Input: part model. Units: mm. Frame: model coordinates. A direction names the side the tool comes from. Round coordinates to 2 decimals unless told otherwise and drop trailing zeros. Loops run counter-clockwise (first coordinate to the right, second up) from the corner with the lowest first, then second, coordinate; pieces in that order, holes last.
(1) Cut plane B-B, the plane y = 4.5. Output: boundary loops of the cut face in (x, z).
(2) Draft query along X for faces 1 (the face through (33.267, -9.491, -9.436)), 2 (the face through (64.422, 8, -4)), 3 (the face through (40.599, -5, -9)). Return one class per face: released by +X, released by -X, zero draft, split by the parting line, or undercut.
(3) First-contact query: pin 1 Ø6 at (x, z) = (59.5, -7.5) entering from -Y; pin 2 Ø1.5 at (x, y) = (44.5, 18.5) entering from +Z; pin 3 Ø1.8 at (y, z) = (-4, -9) entering from -X. Flat tips, straight axial feed; report the tip coordinate or a pass-through.
(4) Line query: line 1 (X direction, y = 4, z = -6.25); line 2 (Y direction, x = 51.5, z = -0.5); line 3 (Z direction, x = 31, y = 7). Output: solid intervals per line, ascending.
(5) Access query for faces 4 (the face through (44, -6.915, -9)), 5 (the face through (44.456, -9.419, -9.436)), 6 (the face through (33, -6.915, -9)), 7 (the face through (13.194, 8, -4)), 8 (the face through (39, -8, -7.62)). Directions: +Z, -Z, +X, -X, +Y, -Y. A direction counts if a zero-diameter tool reaches every point of the face in a straight line with its end or side. Return the directions, or none.
(6) Cut plane A-A, the plane z = -1. Output: boundary loops of the cut face in (x, y).
(7) Cut plane C-C, the plane x = 38.5. Output: boundary loops of the cut face in (y, z) (3 decimals), and give its area (3 significant figures).
(8) Cut plane D-D, the plane x = 30.5. Output: boundary loops of the cut face in (y, z) (3 decimals).
from build123d import *

# Parameters (mm, degrees)
BOSS_EXTRUDE4_DEPTH = 7.62
BOSS_EXTRUDE5_DEPTH = 3.5814
BOSS_EXTRUDE6_DEPTH = 3.5814


with BuildPart() as part:
    # Sketch17 → Boss-Extrude4 (new body)
    with BuildSketch(Plane(origin=(57.616701934, 0, 0), x_dir=(-1, 0, 0), z_dir=(0, 0, -1))):
        Polygon((-9.344833285, -2.54), (-9.344833285, 16.351663206), (2.490045751, 28.186542241), (34.995614796, 28.186542241), (46.962246821, 16.219910216), (46.962246821, -2.54), align=None)
        Polygon((-6.804833285, 0), (-6.804833285, 15.299560757), (3.542148199, 25.646542241), (33.943512348, 25.646542241), (44.422246821, 15.167807768), (44.422246821, 0), align=None, mode=Mode.SUBTRACT)
    extrude(amount=BOSS_EXTRUDE4_DEPTH)

    # Sketch20 → Boss-Extrude5 (add)
    with BuildSketch(Plane(origin=(0, 0, -7.62), x_dir=(-1, 0, 0), z_dir=(0, 0, -1))):
        Polygon((-66.961535219, -2.54), (-66.961535219, 16.351663206), (-55.126656184, 28.186542241), (-22.621087138, 28.186542241), (-10.654455113, 16.219910216), (-10.654455113, -2.54), align=None)
    extrude(amount=BOSS_EXTRUDE5_DEPTH)

    # Sketch21 → Boss-Extrude6 (add)
    with BuildSketch(Plane(origin=(0, 0, -11.2014), x_dir=(-1, 0, 0), z_dir=(0, 0, -1))):
        Polygon((-40.598695166, -6.9149976), (-48.205995166, -6.9149976), (-40.598695166, -11.9949976), (-37.017295166, -11.9949976), (-29.409995166, -6.9149976), (-37.017295166, -6.9149976), (-37.017295166, -2.54), (-40.598695166, -2.54), align=None)
    extrude(amount=-BOSS_EXTRUDE6_DEPTH)


solid = part.part
Reported:
1. outline: (10.65, -11.2) - (66.96, -11.2) - (66.96, 0) - (64.42, 0) - (64.42, -7.62) - (13.19, -7.62) - (13.19, 0) - (10.65, 0) - close
2. face 1: released by -X
2. face 2: undercut
2. face 3: released by +X
3. pin 1: stops at y = -2.54
3. pin 2: stops at z = -7.62
3. pin 3: stops at x = 37.02
4. line 1: x = 10.65 to 13.19, 64.42 to 66.96
4. line 2: y = -2.54 to 0, 25.65 to 28.19
4. line 3: z = -11.2 to -7.62
5. face 4: +Z, -Z, +X
5. face 5: +Z, -Z, +X, -Y
5. face 6: +Z, -Z, -X
5. face 7: +Z
5. face 8: +Z, +X, -X, -Y
6. outline: (10.65, -2.54) - (66.96, -2.54) - (66.96, 16.35) - (55.13, 28.19) - (22.62, 28.19) - (10.65, 16.22) - close; hole (13.19, 0) - (64.42, 0) - (64.42, 15.3) - (54.07, 25.65) - (23.67, 25.65) - (13.19, 15.17) - close
7. outline: (-11.995, -11.201) - (28.187, -11.201) - (28.187, 0) - (25.647, 0) - (25.647, -7.62) - (0, -7.62) - (0, 0) - (-2.54, 0) - (-2.54, -7.62) - (-11.995, -7.62) - close
7. area: 183 mm2
8. outline: (-7.643, -11.201) - (-6.915, -11.201) - (-6.915, -7.62) - (-7.643, -7.62) - close; (-2.54, -11.201) - (28.187, -11.201) - (28.187, 0) - (25.647, 0) - (25.647, -7.62) - (0, -7.62) - (0, 0) - (-2.54, 0) - close
